CAD build for the part. Positions are in the model's coordinates, mm. Face numbers are marked on the shaded views. A direction names the side the tool comes from. Round coordinates to 2 decimals unless told otherwise and drop trailing zeros. Loops run counter-clockwise (first coordinate to the right, second up) from the corner with the lowest first, then second, coordinate; pieces in that order, holes last.
```python
from build123d import *

# Parameters (mm, degrees)
F0_W        = 60
F0_H        = 26
F1_DEPTH    = 5
F2_R        = 11.25
F3_DEPTH    = 8
F4_R        = 11.25
F4_R_2      = 10.7332604818
F5_DEPTH    = 1
F6_SIZE     = 1
F7_W        = 60
F7_H        = 9.3
F8_DEPTH    = 1.9
F9_T4_DEPTH = 70.2867319519
F9_T9_DEPTH = 70.2867319519
F10_W       = 60
F10_H       = 6.5
F11_DEPTH   = 4.1
F12_SIZE    = 0.5
F13_R       = 2.85
F14_DEPTH   = 12.5
F15_W       = 6
F15_H       = 6
F16_DEPTH   = 12.5


# Not quite as in the source:
# - a fillet or chamfer that OpenCascade refuses, or shapes differently, is made with other operations: its cross-section is extruded or revolved along the edge and cut away or added


with BuildPart() as f1:
    # F0 (on Front) → F1 (new body)
    with BuildSketch(Plane.XZ):
        Rectangle(F0_W, F0_H)
    extrude(amount=F1_DEPTH)

    # F2 (on face) → F3 (join)
    with BuildSketch(Plane.XZ.offset(5)):
        with BuildLine():
            ThreePointArc((2.6e-08, -13), (9.1923881646, -9.1923881462), (13, 0))
            ThreePointArc((13, 0), (9.1923881562, 9.1923881546), (2.2e-09, 13))
            ThreePointArc((2.2e-09, 13), (-13, -1.19e-08), (2.6e-08, -13))
        make_face()
        Circle(F2_R, mode=Mode.SUBTRACT)
    extrude(amount=F3_DEPTH)

    # F4 (on face) → F5 (join)
    with BuildSketch(Plane.XZ.offset(5)):
        Circle(F4_R)
        Circle(F4_R_2, mode=Mode.SUBTRACT)
    extrude(amount=F5_DEPTH)

    # F6
    f6_edges = [f1.edges().sort_by_distance(p)[0] for p in [
        (-11.25, -13, 0),
    ]]
    chamfer(f6_edges, length=F6_SIZE)

    # F7 (on face) → F8 (join)
    with BuildSketch(Plane(origin=(0, 0, 0), x_dir=(-1, 0, 0), z_dir=(0, 1, 0))):
        Rectangle(F7_W, F7_H)
    extrude(amount=F8_DEPTH)

    # F9: chamfer of 2 on 2 edges, made by hand


with BuildPart() as f9_tool2:
    # F9_s3 → F9_t4 (new body)
    with BuildSketch(Plane.YZ.offset(-35.1433659759)):
        Polygon((-0.1, 4.65), (1.9, 2.65), (1.9, 4.65), align=None)
    extrude(amount=F9_T4_DEPTH)

    split(bisect_by=Plane.XZ, keep=Keep.BOTTOM)


with BuildPart() as f1_1:
    add(f1.part)

    # F9_t1: cut F9_tool2
    add(f9_tool2.part, mode=Mode.SUBTRACT)


with BuildPart() as f9_tool7:
    # F9_s8 → F9_t9 (new body)
    with BuildSketch(Plane.YZ.offset(35.1433659759)):
        Polygon((-0.1, -4.65), (1.9, -2.65), (1.9, -4.65), align=None)
    extrude(amount=-F9_T9_DEPTH)

    split(bisect_by=Plane.XZ, keep=Keep.BOTTOM)


with BuildPart() as f1_2:
    add(f1_1.part)

    # F9_t6: cut F9_tool7
    add(f9_tool7.part, mode=Mode.SUBTRACT)

    # F10 (on face) → F11 (join)
    with BuildSketch(Plane(origin=(0, 1.9, 0), x_dir=(-1, 0, 0), z_dir=(0, 1, 0))):
        Rectangle(F10_W, F10_H)
    extrude(amount=F11_DEPTH)

    # F12
    f12_edges = [f1_2.edges().sort_by_distance(p)[0] for p in [
        (0, 6, 3.25),
        (0, 6, -3.25),
    ]]
    chamfer(f12_edges, length=F12_SIZE)

    # F13 (on Front) → F14 (cut, symmetric)
    with BuildSketch(Plane.XZ):
        Circle(F13_R)
    extrude(amount=F14_DEPTH, both=True, mode=Mode.SUBTRACT)

    # F15 (on Top) → F16 (cut, symmetric)
    with BuildSketch(Plane.XY):
        with Locations((3, 3)):
            Rectangle(F15_W, F15_H)
        with Locations((-3, 3)):
            Rectangle(F15_W, F15_H)
    extrude(amount=F16_DEPTH, both=True, mode=Mode.SUBTRACT)


solid = f1_2.part
```
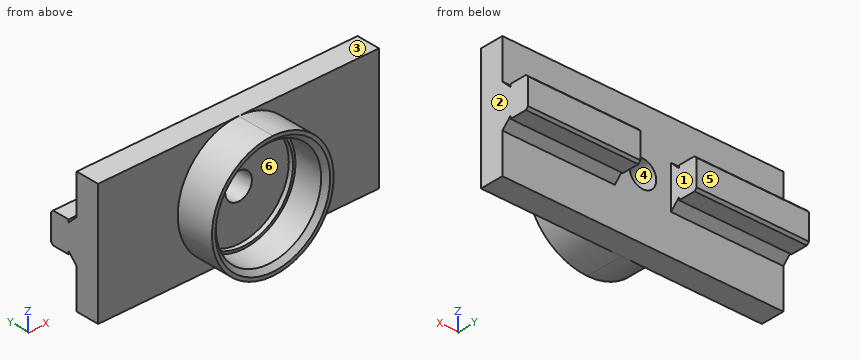
Item 1: Probe line 1 (X direction, y = -1.5, z = 0.25); line 2 (Y direction, x = -23, z = 8.5); line 3 (X direction, y = -9.25, z = -1.75). List the from-to ranges inside material, lowest first.
Answers follow:
line 1: x = -30 to -2.84, 2.84 to 30
line 2: y = -5 to 0
line 3: x = -12.88 to -11.11, 11.11 to 12.88
Item 2: Cut at C-C, the plane y = -2.75. Give the cut face in (x, z).
Answers follow:
outline: (-30, -13) - (30, -13) - (30, 13) - (-30, 13) - close; hole circle Ø5.7 at (0, 0)
Item 3: Two-plate mould, pull along X, no slides. Class the marked faces 1, 2, 3 and 4: released by +X, released by -X, zero draft, split by the parting line, or undercut.
Answers follow:
face 1: undercut
face 2: released by +X
face 3: zero draft
face 4: undercut
Item 4: Flat gauge pins, fed straight in: P1, Ø10, axis at x = 18.5, z = 7, coming from the -Y side; P2, Ø3, axis at x = 24, y = 4, coming from the +Z side; P3, Ø1, axis at y = -6.5, z = 9, coming from the -X side; P4, Ø5, axis at x = 0, z = 0, coming from the +Y side. Where does each tip first touch, or does it go through?
Answers follow:
P1: stops at y = -5
P2: stops at z = 3.25
P3: stops at x = -9.84
P4: passes through
Item 5: Cut at B-B, the plane x = 25. Give the cut face in (y, z), plus the area to 3 significant figures.
Answers follow:
outline: (-5, -13) - (0, -13) - (0, -4.55) - (1.9, -2.65) - (1.9, -3.25) - (5.5, -3.25) - (6, -2.75) - (6, 2.75) - (5.5, 3.25) - (1.9, 3.25) - (1.9, 2.65) - (0, 4.55) - (0, 13) - (-5, 13) - close
area: 170 mm2
Item 6: Cut at A-A, the plane y = 2.5. Give the cut face in (x, z).
Answers follow:
outline: (-30, -3.25) - (-6, -3.25) - (-6, 3.25) - (-30, 3.25) - close; (6, -3.25) - (30, -3.25) - (30, 3.25) - (6, 3.25) - close
Item 7: Cut at D-D, the plane y = -9.75. Give the cut face in (x, z), plus the area to 3 significant figures.
Answers follow:
outline: circle Ø26 at (0, 0); hole circle Ø22.5 at (0, 0)
area: 133 mm2
Item 8: 3-axis set-ups, long thin cutter, end or side, ignore diameter. For the marked faces 5 and 6: which of +Z, -Z, +X, -X, +Y, -Y reach the whole face in a straight line?
Answers follow:
face 5: +Z, -Z, +X, -X, +Y
face 6: -Y
